The listing builds one solid part. Answer for the finished solid, in the listing's coordinates (mm). Coordinates: 2 decimals unless noted, no trailing zeros. Write each loop counter-clockwise with the first axis right and the second up, starting at its lowest first coordinate (ties: lowest second). Pieces come first, ordered by that corner, then holes.
(1) Straight lines are drawn through the part: line 1 (Z direction, x = 38.1, y = 1.2); line 2 (X direction, y = 0.7, z = 6.35); line 3 (X direction, y = 1.75, z = 19.05). For each, find the intervals that lie inside material, in ascending order.
(2) The part is cut by section C-C on x = 38.1. Determine the outline of the cut face in (y, z) (3 decimals).
(3) The part is cut by section A-A on y = 0.8. Determine the outline of the cut face in (x, z), plus the area to 3 significant figures.
(4) The part is cut by section D-D on x = 88.9. Determine the outline of the cut face in (y, z) (3 decimals).
(5) The part is cut by section B-B on z = -38.1. Determine the outline of the cut face in (x, y) (3 decimals).
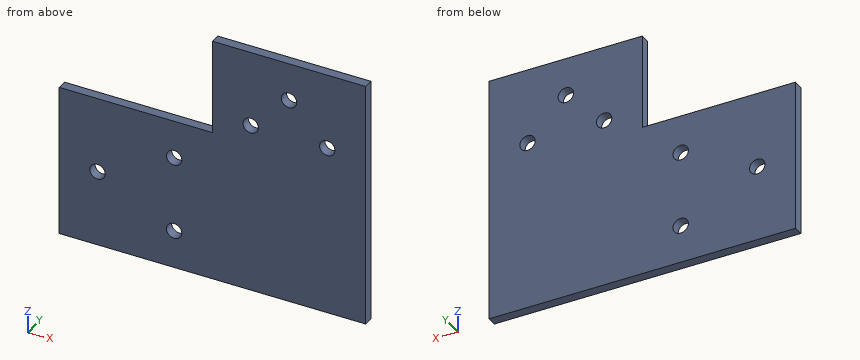
from build123d import *

# Parameters (mm, degrees)
SKETCH1_R           = 2.5527
BOSS_EXTRUDE1_DEPTH = 3.175


with BuildPart() as part:
    # Sketch1 → Boss-Extrude1 (new body)
    with BuildSketch(Plane(origin=(0, 0, 0), x_dir=(1, 0, 0), z_dir=(0, 1, 0))):
        Polygon((0, 0), (50.8, 0), (50.8, -31.75), (101.6, -31.75), (101.6, 50.8), (0, 50.8), align=None)
        with Locations((12.7, 25.4)):
            Circle(SKETCH1_R, mode=Mode.SUBTRACT)
        with Locations((38.1, 12.7)):
            Circle(SKETCH1_R, mode=Mode.SUBTRACT)
        with Locations((38.1, 38.1)):
            Circle(SKETCH1_R, mode=Mode.SUBTRACT)
        with Locations((63.5, -6.35)):
            Circle(SKETCH1_R, mode=Mode.SUBTRACT)
        with Locations((88.9, -6.35)):
            Circle(SKETCH1_R, mode=Mode.SUBTRACT)
        with Locations((76.2, -19.05)):
            Circle(SKETCH1_R, mode=Mode.SUBTRACT)
    extrude(amount=BOSS_EXTRUDE1_DEPTH)


solid = part.part
Model answer:
1. line 1: z = -50.8 to -40.65, -35.55 to -15.25, -10.15 to 0
1. line 2: x = 50.8 to 60.95, 66.05 to 86.35, 91.45 to 101.6
1. line 3: x = 50.8 to 73.65, 78.75 to 101.6
2. outline: (0, -50.8) - (3.175, -50.8) - (3.175, -40.653) - (0, -40.653) - close; (0, -35.547) - (3.175, -35.547) - (3.175, -15.253) - (0, -15.253) - close; (0, -10.147) - (3.175, -10.147) - (3.175, 0) - (0, 0) - close
3. outline: (0, -50.8) - (101.6, -50.8) - (101.6, 31.75) - (50.8, 31.75) - (50.8, 0) - (0, 0) - close; hole circle Ø5.11 at (12.7, -25.4); hole circle Ø5.11 at (38.1, -38.1); hole circle Ø5.11 at (38.1, -12.7); hole circle Ø5.11 at (63.5, 6.35); hole circle Ø5.11 at (76.2, 19.05); hole circle Ø5.11 at (88.9, 6.35)
3. area: 6,650 mm2
4. outline: (0, -50.8) - (3.175, -50.8) - (3.175, 3.797) - (0, 3.797) - close; (0, 8.903) - (3.175, 8.903) - (3.175, 31.75) - (0, 31.75) - close
5. outline: (0, 0) - (35.547, 0) - (35.547, 3.175) - (0, 3.175) - close; (40.653, 0) - (101.6, 0) - (101.6, 3.175) - (40.653, 3.175) - close
